```python
from build123d import *

# Parameters (mm, degrees)
BOSS_EXTRUDE1_DEPTH                = 19.05
M3_CLEARANCE_HOLE1_D               = 3.4
TAPPED_HOLE_FOR_M3X0_5_HELICOIL1_D = 3.15
TAPPED_HOLE_FOR_8_32_HELICOIL1_D   = 4.3942


with BuildPart() as part:
    # Sketch1 → Boss-Extrude1 (new body, symmetric)
    with BuildSketch(Plane(origin=(0, 0, 0), x_dir=(0, 0, -1), z_dir=(1, 0, 0))):
        Polygon((20.6375, 0), (-20.6375, 0), (-20.6375, -16.7005), (-14.2875, -16.7005), (-14.2875, -4.7625), (20.6375, -4.7625), align=None)
    extrude(amount=BOSS_EXTRUDE1_DEPTH, both=True)

    # M3 Clearance Hole1 (through all)
    with Locations(Plane(origin=(0, -4.7625, 0), x_dir=(-1, 0, 0), z_dir=(0, -1, 0))):
        with Locations((-12, 14.2875), (12, 14.2875), (12, -9.7125), (-12, -9.7125)):
            Hole(M3_CLEARANCE_HOLE1_D / 2)

    # Tapped Hole for M3x0.5 Helicoil1 (through all)
    with Locations(Plane(origin=(0, -4.7625, 0), x_dir=(-1, 0, 0), z_dir=(0, -1, 0))):
        with Locations((0, -6.35), (0, 9.525)):
            Hole(TAPPED_HOLE_FOR_M3X0_5_HELICOIL1_D / 2)

    # Tapped Hole for #8-32 Helicoil1 (through all)
    with Locations(Plane.XY.offset(20.6375)):
        with Locations((-11.1125, -8.35025), (11.1125, -8.35025)):
            Hole(TAPPED_HOLE_FOR_8_32_HELICOIL1_D / 2)


solid = part.part
```
Check sheet for the modelled part. Datum: model origin and axes. Units: mm. A direction names the side the tool comes from. Coordinates: 2 decimals unless noted, no trailing zeros. Order: outer loops, then holes, each group sorted by start corner. A loop starts at its lowest first (then second) coordinate and runs counter-clockwise, first axis right, second up. Notation, with made-up numbers: (-20.75, 66.25) -> (-16.75, 66.25) arc R24 cw to (-16.75, 97.25) -> close; hole circle Ø3 at (23.25, 3.5). An arc over 180 degrees is marked (long way). Write each question's results on one line, items separated by ' | '. Start each with the question number.
1) Depth check by flat-ended pin: pin 1 (4.5 mm diameter, centred on x = 12, z = -14.29, fed in from +Y); pin 2 (1 mm diameter, centred on x = 7.5, y = -14, fed in from -Z); pin 3 (10.5 mm diameter, centred on x = 7.5, z = -6.5, fed in from -Y). Enter the tip coordinate at first touch or a pass-through.
2) Section check D-D (x = 11). Enter the section's corners in (y, z), and give its area (3 significant figures).
3) Section check B-B (x = 0). Count the separate pieces of the cut face and the enclosed holes in it, and give its area (3 significant figures).
4) Section check C-C (y = -7). Enter the section's corners in (x, z), and give its area (3 significant figures).
5) Draft check along X on faces 3 (the face through (19.05, -4.5, 4.9)), 4 (the face through (12.784, -2.348, 11.221)), 5 (the face through (0, -16.7, 18)), 6 (the face through (-11.216, -2.348, 11.221)). Enter one of: pulls with the +X half, pulls with the -X half, needs draft (parallel to the pull), parting line crosses it, or undercut.
6) Set-up check for faces 1 (the face through (0, -4.762, -3)), 2 (the face through (11.589, -10.495, 17.418)): record each of +Z, -Z, +X, -X, +Y, -Y from which the full face is reachable in a straight line by a thin tool's end or side.
7) Material ranges on line 1 along Z through (x, y) = (-12, -2.2); line 2 along Y through (x, z) = (-6.5, 8.5); line 3 along X through (y, z) = (-4.5, 7.5), recorded low to high.
Checked values:
1) pin 1: y = 0 | pin 2: z = 14.29 | pin 3: y = -4.76
2) outline: (-16.7, 14.29) -> (-10.54, 14.29) -> (-10.54, 20.64) -> (-16.7, 20.64) -> close; (-6.16, 14.29) -> (-4.76, 14.29) -> (-4.76, 11.09) -> (0, 11.09) -> (0, 20.64) -> (-6.16, 20.64) -> close; (-4.76, -20.64) -> (0, -20.64) -> (0, -15.66) -> (-4.76, -15.66) -> close; (-4.76, -12.91) -> (0, -12.91) -> (0, 8.34) -> (-4.76, 8.34) -> close | area: 218 mm²
3) separate pieces: 3 | enclosed holes: 0 | area: 242 mm²
4) outline: (-19.05, 14.29) -> (-12.85, 14.29) -> (-12.85, 20.64) -> (-19.05, 20.64) -> close; (-9.38, 14.29) -> (9.38, 14.29) -> (9.38, 20.64) -> (-9.38, 20.64) -> close; (12.85, 14.29) -> (19.05, 14.29) -> (19.05, 20.64) -> (12.85, 20.64) -> close | area: 198 mm²
5) face 3: pulls with the +X half | face 4: undercut | face 5: needs draft | face 6: undercut
6) face 1: -Z, +X, -X, -Y | face 2: +Z, -Z
7) line 1: -20.64 to -15.99, -12.59 to 8.01, 11.41 to 20.64 | line 2: -4.76 to 0 | line 3: -19.05 to -1.08, 1.08 to 19.05
